Here's the drawing with two shaded views (mm, measured from the low corner). I have some questions. Coordinates: 2 decimals unless noted, no trailing zeros. Write each loop counter-clockwise with the first axis right and the second up, starting at its lowest first coordinate (ties: lowest second). Pieces come first, ordered by that corner, then holes.
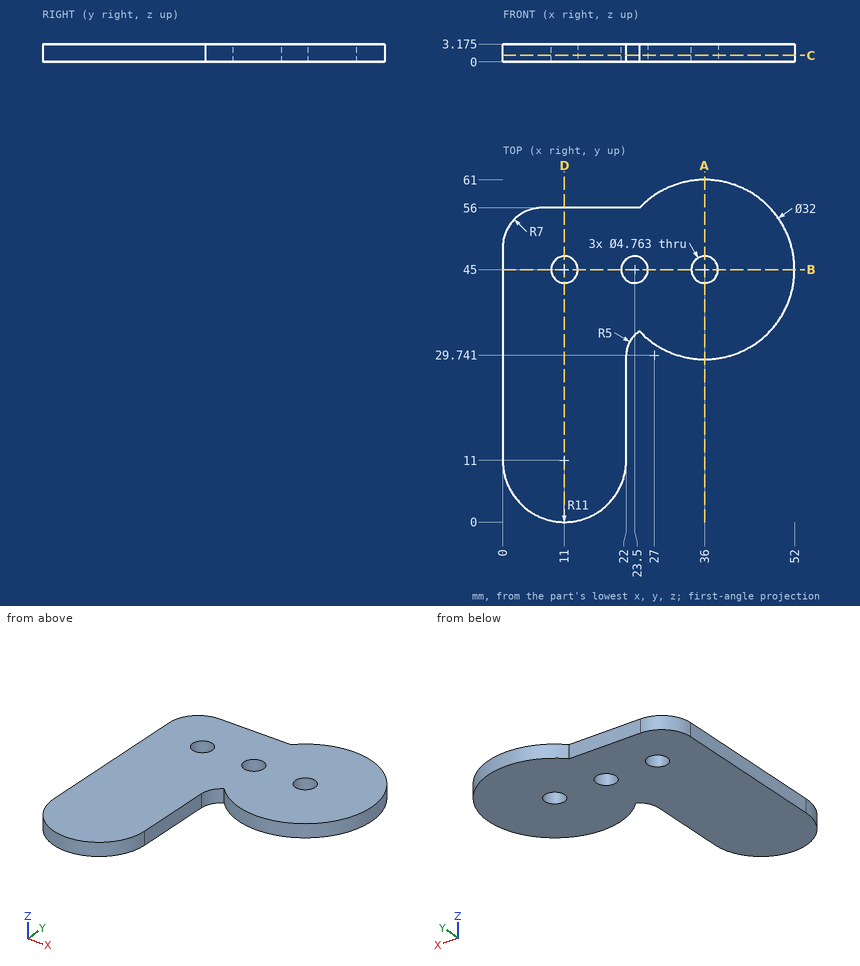
Item 1: If I drill on line 1 along Y through (x, z) = (11, 1.5); line 2 along Y through (x, z) = (23.5, 2.3); line 3 along X through (y, z) = (15, 0.25), over which ranges is the centre line in solid material (lowest first)?
Item 2: I want a section at B-B, the plane y = 45. List the corners of the cut face in (x, z) for me (1 decimal), then the cut area to 3 significant figures.
Item 3: I want a section at D-D, the plane x = 11. List the corners of the cut face in (y, z) for me (1 decimal).
Item 4: Will these pins go through, and if not, where does the flat tip stop? pin 1 Ø1 at (x, z) = (18, 1) entering from +Y; pin 2 Ø1 at (x, z) = (40, 1) entering from +Y; pin 3 Ø1.6 at (y, z) = (17, 2.5) entering from +X.
Item 5: I want a section at A-A, the plane x = 36. List the corners of the cut face in (y, z) for me (1 decimal).
Item 6: I want a section at C-C, the plane z = 1.15. List the corners of the cut face in (x, y) for me, then the cut area to 3 significant figures.
Taken from the geometry:
1. line 1: y = 0 to 42.62, 47.38 to 56
1. line 2: y = 33.31 to 42.62, 47.38 to 56
1. line 3: x = 0 to 22
2. outline: (0, 0) - (8.6, 0) - (8.6, 3.2) - (0, 3.2) - close; (13.4, 0) - (21.1, 0) - (21.1, 3.2) - (13.4, 3.2) - close; (25.9, 0) - (33.6, 0) - (33.6, 3.2) - (25.9, 3.2) - close; (38.4, 0) - (52, 0) - (52, 3.2) - (38.4, 3.2) - close
2. area: 120 mm2
3. outline: (0, 0) - (42.6, 0) - (42.6, 3.2) - (0, 3.2) - close; (47.4, 0) - (56, 0) - (56, 3.2) - (47.4, 3.2) - close
4. pin 1: stops at y = 56
4. pin 2: stops at y = 60.61
4. pin 3: stops at x = 22
5. outline: (29, 0) - (42.6, 0) - (42.6, 3.2) - (29, 3.2) - close; (47.4, 0) - (61, 0) - (61, 3.2) - (47.4, 3.2) - close
6. outline: (0, 11) arc R11 ccw to (22, 11) - (22, 29.74) arc R5 cw to (24.38, 34) arc R16 ccw (long way) to (24.38, 56) - (7, 56) arc R7 ccw to (0, 49) - close; hole circle Ø4.76 at (11, 45); hole circle Ø4.76 at (23.5, 45); hole circle Ø4.76 at (36, 45)
6. area: 1,910 mm2
